from build123d import *

# Parameters (mm, degrees)
F1_DEPTH = 5
F0_R     = 1.5
F2_DEPTH = 3.5
F3_DEPTH = 1
F4_R     = 2


# Not quite as in the source:
# - a feature names something its author has since deleted; it is built from what else it names


with BuildPart() as f1:
    # F0 (on Top) → F1 (new body)
    with BuildSketch(Plane.XY):
        Polygon((35, 36), (14, 36), (-14, 36), (-35, 36), (-35, -36), (35, -36), (35, -33), (35, 33), align=None)
        Polygon((-32, 14.5), (-32, 33), (32, 33), (32, -2), (32, -12.5), (32, -33), (12.7135775983, -33), (-8, -33), (-32, -33), (-32, -14), (-32, 10.5), align=None, mode=Mode.SUBTRACT)
    extrude(amount=F1_DEPTH)



with BuildPart() as f1b:
    # F0 (on Top) → F1, piece 2 (new body)
    with BuildSketch(Plane.XY):
        with BuildLine():
            ThreePointArc((0, 40.5505102572), (5.7267021942, 41.6441264992), (2.5, 46.5))
            ThreePointArc((2.5, 46.5), (1.1441264992, 46.2267021942), (0, 45.4494897428))
            ThreePointArc((0, 45.4494897428), (-1.1441264992, 46.2267021942), (-2.5, 46.5))
            ThreePointArc((-2.5, 46.5), (-5.7267021942, 41.6441264992), (0, 40.5505102572))
        make_face()
        with Locations((-2.5, 43)):
            Circle(F0_R, mode=Mode.SUBTRACT)
        with Locations((2.5, 43)):
            Circle(F0_R, mode=Mode.SUBTRACT)
    extrude(amount=F1_DEPTH)


with BuildPart() as f1_1:
    add(f1.part)

    add(f1b.part)  # F2 merges F1b
    # F0 (on Top) → F2 (join)
    with BuildSketch(Plane.XY):
        with BuildLine():
            Line((-14, 36), (14, 36))
            ThreePointArc((14, 36), (10.4644660941, 37.4644660941), (9, 41))
            Line((9, 41), (9, 46.5))
            Line((9, 46.5), (2.5, 46.5))
            ThreePointArc((2.5, 46.5), (5.7267021942, 41.6441264992), (0, 40.5505102572))
            ThreePointArc((0, 40.5505102572), (-5.7267021942, 41.6441264992), (-2.5, 46.5))
            Line((-2.5, 46.5), (-9, 46.5))
            Line((-9, 46.5), (-9, 41))
            ThreePointArc((-9, 41), (-10.4644660941, 37.4644660941), (-14, 36))
        make_face()
        with BuildLine():
            ThreePointArc((0, 45.4494897428), (1.1441264992, 46.2267021942), (2.5, 46.5))
            Line((2.5, 46.5), (-2.5, 46.5))
            ThreePointArc((-2.5, 46.5), (-1.1441264992, 46.2267021942), (0, 45.4494897428))
        make_face()
    extrude(amount=F2_DEPTH)

    # F0 (on Top) → F3 (join)
    with BuildSketch(Plane.XY):
        Polygon((32, 33), (-32, 33), (-32, 14.5), (-32, 10.5), (-32, -14), (-32, -33), (-8, -33), (12.7135775983, -33), (32, -33), (32, -12.5), (32, -2), align=None)
    extrude(amount=F3_DEPTH)

    # F4
    f4_edges = [f1_1.edges().sort_by_distance(p)[0] for p in [
        (-35, -36, 2.5),
        (35, -36, 2.5),
        (-35, 36, 2.5),
        (35, 36, 2.5),
    ]]
    fillet(f4_edges, radius=F4_R)


solid = f1_1.part
The model under review builds one solid part; all positions refer to its coordinate system, in mm. A direction names the side the tool comes from. Round coordinates to 2 decimals unless told otherwise and drop trailing zeros. Loops run counter-clockwise (first coordinate to the right, second up) from the corner with the lowest first, then second, coordinate; pieces in that order, holes last. Notation, with made-up numbers: M 38,-15.5 L 48,-15.5 A32 ccw 48,11.5 Z; hole C 51.25,28 d6. An arc over 180 degrees is marked long. Answer as a JSON object with one key per item and string values.
Item 1: We need section B-B, the plane z = 2.6. State the section outline as (x, y) points.
Check sheet entries:
{"outline": "M -35,-34 A2 ccw -33,-36 L 33,-36 A2 ccw 35,-34 L 35,34 A2 ccw 33,36 L 14,36 A5 cw 9,41 L 9,46.5 L -9,46.5 L -9,41 A5 cw -14,36 L -33,36 A2 ccw -35,34 Z; hole M -32,-33 L 32,-33 L 32,33 L -32,33 Z; hole C -2.5,43 d3; hole C 2.5,43 d3"}
Item 2: The part is to be moulded in two halves that separate along X. For faces 1 (the face through (32, 0, 3)), 2 (the face through (-35, 0, 2)), 3 (the face through (0, 6, 0)), 4 (the face through (11, 37, 2)), say which applies: +X half, -X half, draft (parallel to the pull), parting line (faces both ways), or undercut.
Check sheet entries:
{"face 1": "undercut", "face 2": "-X half", "face 3": "draft", "face 4": "+X half"}
Item 3: We need section A-A, the plane y = 43. State the section outline as (x, z) points.
Check sheet entries:
{"outline": "M -9,0 L -4,0 L -4,5 L -6,5 L -6,3.5 L -9,3.5 Z; M -1,0 L 1,0 L 1,5 L -1,5 Z; M 4,0 L 9,0 L 9,3.5 L 6,3.5 L 6,5 L 4,5 Z"}
Item 4: For line 1 along Y through (x, z) = (2.5, 2.5); line 2 along X through (y, z) = (7, 2.85); line 3 along Y through (x, z) = (21.5, 4.1), list the stretches that pass through material, from the lowest coordinate up.
Check sheet entries:
{"line 1": "-36 to -33, 33 to 41.5, 44.5 to 46.5", "line 2": "-35 to -32, 32 to 35", "line 3": "-36 to -33, 33 to 36"}
Item 5: Tool access review of faces 5 (the face through (0, 0, 1)), 6 (the face through (-9, 44, 2)), 7 (the face through (-34.43, -35.4, 2.54)), 8 (the face through (-34, 0, 5)), 9 (the face through (9, 44, 2)): name each direction out of +Z, -Z, +X, -X, +Y, -Y from which nothing blocks a thin tool from reaching the whole face with its end or side.
Check sheet entries:
{"face 5": "+Z", "face 6": "+Z, -Z, -X, +Y", "face 7": "+Z, -Z, -X, -Y", "face 8": "+Z, +X, -X, +Y, -Y", "face 9": "+Z, -Z, +X, +Y"}
Item 6: We need section D-D, the plane y = -19. State the section outline as (x, z) points, and give its area (3 significant figures).
Check sheet entries:
{"outline": "M -35,0 L 35,0 L 35,5 L 32,5 L 32,1 L -32,1 L -32,5 L -35,5 Z", "area": "94.0 mm2"}
Item 7: Clearance check with flat-ended pins moving along their axes: P1, Ø2.5, axis at x = 2.5, y = 43, coming from the +Z side; P2, Ø1, axis at x = -23.5, y = -3, coming from the +Z side; P3, Ø1, axis at y = 44.5, z = 2, coming from the +X side. State where each tip first meets the part, or that it passes through.
Check sheet entries:
{"P1": "through", "P2": "z = 1", "P3": "x = 9"}
Item 8: We need section C-C, the plane x = -31. State the section outline as (y, z) points.
Check sheet entries:
{"outline": "M -36,0 L 36,0 L 36,5 L 33,5 L 33,1 L -33,1 L -33,5 L -36,5 Z"}
